The model under review builds one solid part; all positions refer to its coordinate system, in mm. Round coordinates to 2 decimals unless told otherwise and drop trailing zeros. Loops run counter-clockwise (first coordinate to the right, second up) from the corner with the lowest first, then second, coordinate; pieces in that order, holes last. Notation, with made-up numbers: (2, -27.75) - (29, -27.75) arc R21 cw to (29, -23.75) - close; hole circle Ø4 at (82, -29). An arc over 180 degrees is marked (long way). Answer as CSV lines item,"result".
from build123d import *

# Parameters (mm, degrees)
ESBO_O1_R                = 14
RESSALTO_EXTRUS_O1_DEPTH = 0.1


with BuildPart() as part:
    # Esboço1 → Ressalto-extrusão1 (new, symmetric)
    with BuildSketch(Plane(origin=(0, 0, 0), x_dir=(1, 0, 0), z_dir=(0, 1, 0))):
        Polygon((-7.05, 19.55), (-8.097875144, 19.55), (-19.55, 8.097875144), (-19.55, -8.097875144), (-8.097875144, -19.55), (8.097875144, -19.55), (19.55, -8.097875144), (19.55, 8.097875144), (8.097875144, 19.55), (7.05, 19.55), (7.05, 23.85), (-7.05, 23.85), align=None)
        with Locations(Location((0, 0, 0), (0, 0, 270))):
            Circle(ESBO_O1_R, mode=Mode.SUBTRACT)
    extrude(amount=RESSALTO_EXTRUS_O1_DEPTH, both=True)


solid = part.part
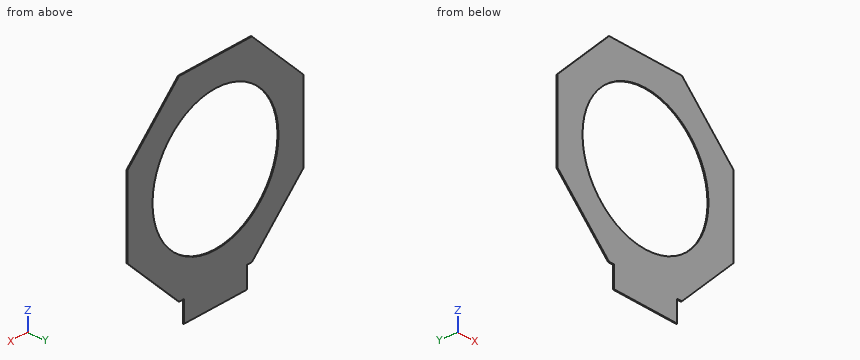
1. Take a section at C-C (y = 0.05). State the section outline as (x, z) points.
Numbers:
outline,"(-19.55, -8.1) - (-8.1, -19.55) - (-7.05, -19.55) - (-7.05, -23.85) - (7.05, -23.85) - (7.05, -19.55) - (8.1, -19.55) - (19.55, -8.1) - (19.55, 8.1) - (8.1, 19.55) - (-8.1, 19.55) - (-19.55, 8.1) - close; hole circle Ø28 at (0, 0)"
2. Wall thickness on probe 1 along X at (y, z) = (0, 0); probe 2 along X at (y, z) = (0, -9); probe 3 along Z at (x, y) = (8, 0.05): over which ranges is each line inside the solid? List them lowest first.
Numbers:
probe 1,"x = -19.55 to -14, 14 to 19.55"
probe 2,"x = -18.65 to -10.72, 10.72 to 18.65"
probe 3,"z = -19.55 to -11.49, 11.49 to 19.55"
3. Take a section at A-A (x = 0). State the section outline as (y, z) points.
Numbers:
outline,"(-0.1, -23.85) - (0.1, -23.85) - (0.1, -14) - (-0.1, -14) - close; (-0.1, 14) - (0.1, 14) - (0.1, 19.55) - (-0.1, 19.55) - close"
4. Take a section at B-B (z = 0). State the section outline as (x, y) points.
Numbers:
outline,"(-19.55, -0.1) - (-14, -0.1) - (-14, 0.1) - (-19.55, 0.1) - close; (14, -0.1) - (19.55, -0.1) - (19.55, 0.1) - (14, 0.1) - close"
5. Take a section at D-D (z = 16.5). State the section outline as (x, y) points.
Numbers:
outline,"(-11.15, -0.1) - (11.15, -0.1) - (11.15, 0.1) - (-11.15, 0.1) - close"
